from build123d import *

# Parameters (mm, degrees)
SKETCH_1_W      = 10
SKETCH_1_H      = 5
EXTRUDE_1_DEPTH = 5
SKETCH_1_3_W    = 10
SKETCH_1_3_H    = 5
EXTRUDE_2_DEPTH = 10
EXTRUDE_3_DEPTH = 15


with BuildPart() as part:
    # Sketch 1 → Extrude 1 (new body)
    with BuildSketch(Plane(origin=(0, 0, 0), x_dir=(1, 0, 0), z_dir=(0, 1, 0))):
        Polygon((5, 5), (-5, 5), (-5, -5), (5, -5), (5, -10), (15, -10), (15, 10), (5, 10), align=None)
        with Locations((0, -7.5)):
            Rectangle(SKETCH_1_W, SKETCH_1_H)
        Polygon((-5, 5), (-5, 10), (-15, 10), (-15, -10), (-5, -10), (-5, -5), align=None)
        with Locations((0, 7.5)):
            Rectangle(SKETCH_1_W, SKETCH_1_H)
    extrude(amount=EXTRUDE_1_DEPTH)

    # Sketch 1_3 → Extrude 2 (add)
    with BuildSketch(Plane(origin=(0, 0, 0), x_dir=(1, 0, 0), z_dir=(0, 1, 0))):
        with Locations((0, 7.5)):
            Rectangle(SKETCH_1_3_W, SKETCH_1_3_H)
        with Locations((0, -7.5)):
            Rectangle(SKETCH_1_3_W, SKETCH_1_3_H)
        Polygon((-5, 5), (-5, 10), (-15, 10), (-15, -10), (-5, -10), (-5, -5), align=None)
    extrude(amount=EXTRUDE_2_DEPTH)

    # Sketch 1_4 → Extrude 3 (add)
    with BuildSketch(Plane(origin=(0, 0, 0), x_dir=(1, 0, 0), z_dir=(0, 1, 0))):
        Polygon((-5, 5), (-5, 10), (-15, 10), (-15, -10), (-5, -10), (-5, -5), align=None)
    extrude(amount=EXTRUDE_3_DEPTH)


solid = part.part
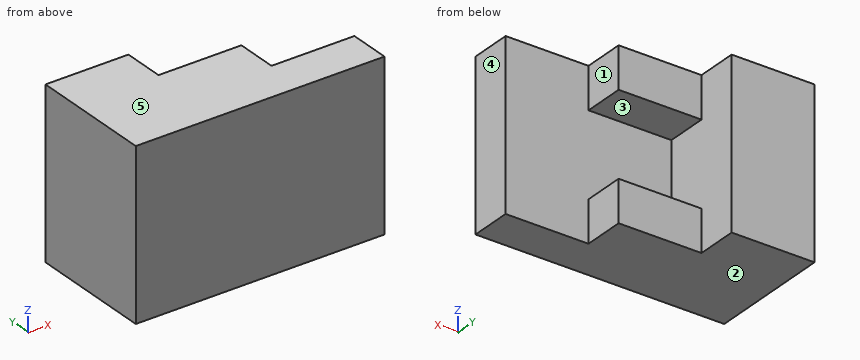
Work out the finished part from the listing and answer in its coordinate system (mm). Face numbers are marked on the shaded views. A direction names the side the tool comes from. Give positions to 0.01 mm unless a question says otherwise; leave off trailing zeros. Order: outer loops, then holes, each group sorted by start corner. A loop starts at its lowest first (then second) coordinate and runs counter-clockwise, first axis right, second up. Notation, with made-up numbers: (41, 16) - (57, 16) arc R22 cw to (57, 51) - close; hole circle Ø11 at (80, 10.25). An arc over 180 degrees is marked (long way). Answer as CSV lines item,"result". Start each with the question number.
Q1. The part is cut by section A-A (z = -3.75). Write down the section's boundary in (x, y).
Q2. The part is cut by section D-D (y = 12.25). Write down the section's boundary in (x, z).
Q3. Given pin 1 Ø3 at (y, z) = (8, 1) entering from +X; pin 2 Ø1 at (x, z) = (1, 3.5) entering from +Y; pin 3 Ø4 at (x, z) = (2, -7) entering from +Y; pin 4 Ø1.5 at (x, y) = (10, 5.5) entering from +Z, each flat-ended and moving along its own axis, determine where each tip first touches the part or whether it passes through.
Q4. The part is cut by section B-B (y = 5.5). Write down the section's boundary in (x, z), then the cut area to 3 significant figures.
Q5. The part is cut by section C-C (x = 0). Write down the section's boundary in (y, z), then the cut area to 3 significant figures.
Q6. The mould has two halves that part along Z. Classify the marked faces 3, 4 and 5: +Z half, -Z half, draft (parallel to the pull), parting line (faces both ways), or undercut.
Q7. Find the intervals of material crossed by L1, parallel to Z at x = -3.75, y = 9.25; L2, parallel to Y at x = 11.5, z = 5.25; L3, parallel to X at y = 8, z = -8, in increasing order. Write a range as [from, to].
Q8. For the marked faces 1 and 2, determine the directions among +Z, -Z, +X, -X, +Y, -Y from which every point of the face is accessible in a straight line to the end or side of a thin tool.
Check result:
1,outline,"(-15, 0) - (15, 0) - (15, 5) - (-5, 5) - (-5, 15) - (-15, 15) - close"
2,outline,"(-15, -10) - (-5, -10) - (-5, 10) - (-15, 10) - close"
3,pin 1,"stops at x = -5"
3,pin 2,"stops at y = 5"
3,pin 3,"stops at y = 10"
3,pin 4,"stops at z = 10"
4,outline,"(-15, -10) - (5, -10) - (5, -5) - (-5, -5) - (-5, 5) - (5, 5) - (5, 10) - (-15, 10) - close"
4,area,"300 mm²"
5,outline,"(0, -10) - (10, -10) - (10, -5) - (5, -5) - (5, 5) - (10, 5) - (10, 10) - (0, 10) - close"
5,area,"150 mm²"
6,face 3,"undercut"
6,face 4,"draft"
6,face 5,"+Z half"
7,L1,"z = [-10, -5], [5, 10]"
7,L2,"y = [0, 5]"
7,L3,"x = [-15, 5]"
8,face 1,"+Z, -Z, +X, +Y"
8,face 2,"-Z, +X, -X, +Y, -Y"
